Design review of the part built by this model. Coordinates are the model's own, in mm. Give positions to 0.01 mm unless a question says otherwise; leave off trailing zeros. Loops run counter-clockwise (first coordinate to the right, second up) from the corner with the lowest first, then second, coordinate; pieces in that order, holes last. Notation, with made-up numbers: (2, 70) -> (12, 70) arc R4 cw to (12, 75) -> close; hole circle Ø10 at (-13, 49.25). An arc over 180 degrees is marked (long way). Use a Markdown table: item, result. Add a question column.
1. To check wall thickness, follow line 1 (Y direction, x = 0, z = 54); line 2 (Y direction, x = 38, z = 41.5); line 3 (X direction, y = 27.5, z = 38). State the ranges of each line that lie inside material, in increasing order.
2. Draft analysis for pull direction X (two halves, no side actions). For faces 1 (the flat face through (-22, 44, 76.2)), 2 (the cylindrical face through (-12.779, -57.547, 37.567)), 3 (the cylindrical face through (46.717, 14.712, 37.567)), state which applies: pulls with the +X half, pulls with the -X half, needs draft (parallel to the pull), parting line crosses it, or undercut.
3. For pin 1 Ø12 at (y, z) = (-31, 57.5) entering from -X; pin 2 Ø10 at (x, z) = (-31.5, 44) entering from +Y; pin 3 Ø8 at (x, z) = (0.5, 53) entering from -Y, all flat-tipped, find the tip position at first contact; note any pin that passes through.
4. Add section C-C (z = 69). State the section outline as (x, y) points, and give its area (3 significant figures).
5. Add section A-A (x = 0). State the section outline as (y, z) points.
```python
from build123d import *

# Parameters (mm, degrees)
F0_R     = 58.9489571111
F0_R_2   = 48.9787868108
F1_DEPTH = 25.4
F2_DEPTH = 25.4
F3_DEPTH = 25.4


with BuildPart() as f1:
    # F0 (on Top) → F1 (new body)
    with BuildSketch(Plane.XY):
        Circle(F0_R)
        Circle(F0_R_2, mode=Mode.SUBTRACT)
    extrude(amount=F1_DEPTH)

    # F2 (add): faces of the model
    f2_faces = [f1.faces().sort_by_distance(p)[0] for p in [
        (-57.2816288184, 0, 25.4),
        (-57.2816288184, 0, 0),
    ]]
    extrude(f2_faces, amount=F2_DEPTH, dir=(0, 0, 1))

    # F3 (add): a face of the model
    f3_faces = [f1.faces().sort_by_distance(p)[0] for p in [
        (-57.2816288184, 0, 50.8),
    ]]
    extrude(f3_faces, amount=F3_DEPTH)


solid = f1.part
```
Taken from the geometry:
| question | item | result |
|---|---|---|
| 1 | line 1 | y = -58.95 to -48.98, 48.98 to 58.95 |
| 1 | line 2 | y = -45.07 to -30.9, 30.9 to 45.07 |
| 1 | line 3 | x = -52.14 to -40.53, 40.53 to 52.14 |
| 2 | face 1 | needs draft |
| 2 | face 2 | parting line crosses it |
| 2 | face 3 | undercut |
| 3 | pin 1 | stops at x = -53.39 |
| 3 | pin 2 | stops at y = 52.66 |
| 3 | pin 3 | stops at y = -58.95 |
| 4 | outline | circle Ø117.9 at (0, 0); hole circle Ø97.96 at (0, 0) |
| 4 | area | 3,380 mm^2 |
| 5 | outline | (-58.95, 0) -> (-48.98, 0) -> (-48.98, 76.2) -> (-58.95, 76.2) -> close; (48.98, 0) -> (58.95, 0) -> (58.95, 76.2) -> (48.98, 76.2) -> close |
